```python
from build123d import *

# Parameters (mm, degrees)
BASPROSKE_W        = 6
BASPROSKE_H        = 4.5
TOOTHCUT_DEPTH     = 9.746427842
TEETHCUTS_COUNT    = 13
CUT_EXTRUDE1_REACH = 10.736


with BuildPart() as part:
    # BasProSke → Base-Revolve (revolve)
    with BuildSketch(Plane(origin=(0, 0, 0), x_dir=(1, 0, 0), z_dir=(0, 1, 0)), mode=Mode.PRIVATE) as base_revolve_sk:
        with Locations((3, 2.25)):
            Rectangle(BASPROSKE_W, BASPROSKE_H)
    revolve(base_revolve_sk.sketch.rotate(Axis((-10, 0, 0), (1, 0, 0)), 180), axis=Axis((-10, 0, 0), (1, 0, 0)))

    # TooCutSke → ToothCut (cut, through all)
    with BuildSketch(Plane(origin=(0, 0, 0), x_dir=(0, 0, -1), z_dir=(1, 0, 0))):
        with BuildLine():
            ThreePointArc((0.330578579, 3.131600039), (0, 3.149), (-0.330578579, 3.131600039))
            ThreePointArc((-0.330578579, 3.131600039), (-0.504119116, 3.854627805), (-0.992642471, 4.415190379))
            ThreePointArc((-0.992642471, 4.415190379), (0, 4.5254), (0.992642471, 4.415190379))
            ThreePointArc((0.992642471, 4.415190379), (0.504119116, 3.854627805), (0.330578579, 3.131600039))
        make_face()
    toothcut = extrude(amount=TOOTHCUT_DEPTH, mode=Mode.SUBTRACT)

    # TeethCuts: ToothCut ×13 about axis
    teethcuts_axis = Axis((0, 0, 0), (1, 0, 0))
    for i in range(1, TEETHCUTS_COUNT):
        add(toothcut.rotate(teethcuts_axis, i * 360 / TEETHCUTS_COUNT), mode=Mode.SUBTRACT)

    # Sketch1 → Cut-Extrude1 (cut, up to next)
    with BuildSketch(Plane.ZY, mode=Mode.PRIVATE) as cut_extrude1_sk1:
        with BuildLine():
            Line((-1.05, 1.035917468), (-1.05, -1.035917468))
            ThreePointArc((-1.05, -1.035917468), (1.475, 0), (-1.05, 1.035917468))
        make_face()
    cut_extrude1_tool1 = extrude(cut_extrude1_sk1.sketch, amount=-CUT_EXTRUDE1_REACH, mode=Mode.PRIVATE) & part.part
    add(cut_extrude1_tool1.solids().sort_by_distance((0, 0, 0.118985))[0], mode=Mode.SUBTRACT)


solid = part.part
```
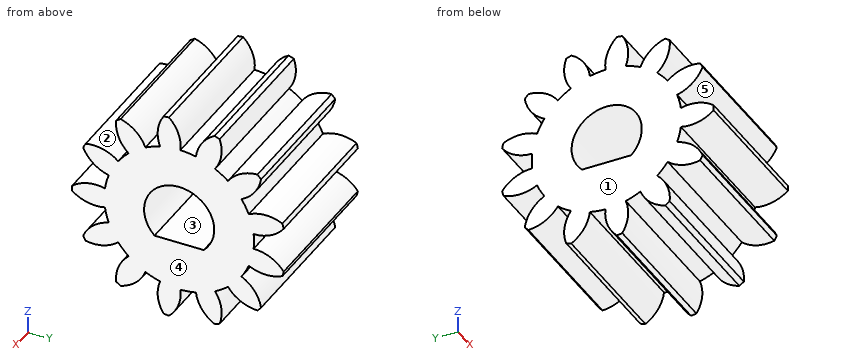
Input: part model. Units: mm. Frame: model coordinates. Face numbers are marked on the shaded views. A direction names the side the tool comes from. Coordinates: 2 decimals unless noted, no trailing zeros. Write each loop counter-clockwise with the first axis right and the second up, starting at its lowest first coordinate (ties: lowest second). Pieces come first, ordered by that corner, then holes. Notation, with made-up numbers: (60, -34.75) -> (89, -34.75) arc R27 cw to (89, -4.75) -> close; hole circle Ø8 at (18.5, 56). An arc over 180 degrees is marked (long way). Answer as a JSON object with one key per item and string values.
1. Mould query, pull axis Y, two halves, no side actions, for the marked faces 1 and 2. Classes: released by +Y, released by -Y, zero draft, split by the parting line, or undercut.
Result set:
{"face 1": "zero draft", "face 2": "undercut"}
2. Section B-B on y = 2.5. Return the cut outline in (x, z).
Result set:
{"outline": "(0, -2.82) -> (6, -2.82) -> (6, 2.82) -> (0, 2.82) -> close"}
3. Material intervals for line 1 (Y direction, x = 0.8, z = 0) (3 decimals); line 2 (Z direction, x = 1.95, y = -2.5); line 3 (Z direction, x = 0.4, y = -3.25), sorted ascending. Write a range as from..to.
Result set:
{"line 1": "y = -4.5..-1.475, 1.475..3.149", "line 2": "z = -3.74..-2.82, -1.91..1.91, 2.82..3.74", "line 3": "z = -2.19..-1.17, -0.46..0.46, 1.17..2.19"}
4. First-contact query: P1, Ø1, axis at x = 4, z = -2, coming from the +Y side. Flat tip, straight axial feed; report the tip coordinate or a pass-through.
Result set:
{"P1": "stops at y = 3.33"}
5. Access query for the marked faces 3, 4 and 5. Directions: +Z, -Z, +X, -X, +Y, -Y. A direction counts if a zero-diameter tool reaches every point of the face in a straight line with its end or side. Return the directions, or none.
Result set:
{"face 3": "+X, -X", "face 4": "+Z, -Z, +X, +Y, -Y", "face 5": "+X, -X, -Y"}
6. Section A-A on z = 0. Return the cut outline in (x, y) (3 decimals), then the cut area to 3 significant figures.
Result set:
{"outline": "(0, -4.5) -> (6, -4.5) -> (6, -1.475) -> (0, -1.475) -> close; (0, 1.475) -> (6, 1.475) -> (6, 3.149) -> (0, 3.149) -> close", "area": "28.2 mm2"}
